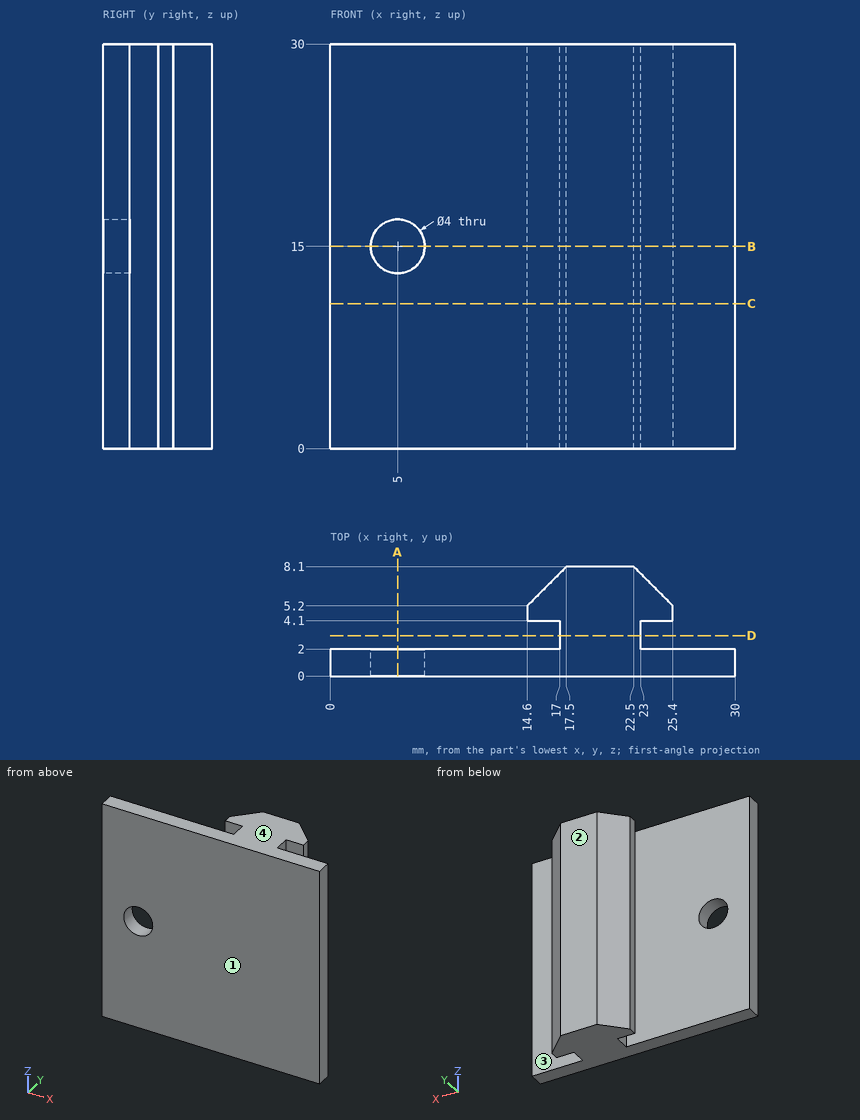
Study the drawing (mm; zero at the part's minimum x, y, z) and answer. Give positions to 0.01 mm unless a question says otherwise; leave off trailing zeros. Loops run counter-clockwise (first coordinate to the right, second up) from the corner with the lowest first, then second, coordinate; pieces in that order, holes last. Notation, with made-up numbers: M -6.5,-37.5 L 33.5,-37.5 A30 ccw 33.5,-12.5 Z; hole C -0.75,12 d7. An arc over 180 degrees is marked long. One line per item, written item: value. Start each with the question number.
1. Find section A-A (x = 5). Give the vertices of the cut face in (y, z).
2. Each of these flat-tipped pins is pushed along its axis until it touches: P1, Ø1.2, axis at y = 4.5, z = 9.5, coming from the -X side; P2, Ø5, axis at x = 5, z = 21, coming from the +Y side; P3, Ø0.6, axis at y = 3, z = 21.5, coming from the +X side. Where does it stop, or does it pass through?
3. Find section B-B (z = 15). Give the vertices of the cut face in (x, y), and give its area (3 significant figures).
4. Find the intervals of material crossed by probe 1 along Z at (x, y) = (5, 1.25); probe 2 along X at (y, z) = (1.3, 15); probe 3 along X at (y, z) = (4.5, 26.25), in increasing order.
5. Find section D-D (y = 3). Give the vertices of the cut face in (x, z).
6. Find section C-C (z = 10.75). Give the vertices of the cut face in (x, y).
7. Determine the mould class of the marked faces 1, 2, 3 and 4 for opening direction Y: released by +Y, released by -Y, zero draft, split by the parting line, or undercut.
Reported:
1. outline: M 0,0 L 2,0 L 2,13 L 0,13 Z; M 0,17 L 2,17 L 2,30 L 0,30 Z
2. P1: stops at x = 14.6
2. P2: stops at y = 2
2. P3: stops at x = 23
3. outline: M 0,0 L 3,0 L 3,2 L 0,2 Z; M 7,0 L 30,0 L 30,2 L 23,2 L 23,4.1 L 25.4,4.1 L 25.4,5.2 L 22.5,8.1 L 17.5,8.1 L 14.6,5.2 L 14.6,4.1 L 17,4.1 L 17,2 L 7,2 Z
3. area: 99.4 mm²
4. probe 1: z = 0 to 13, 17 to 30
4. probe 2: x = 0 to 3, 7 to 30
4. probe 3: x = 14.6 to 25.4
5. outline: M 17,0 L 23,0 L 23,30 L 17,30 Z
6. outline: M 0,0 L 30,0 L 30,2 L 23,2 L 23,4.1 L 25.4,4.1 L 25.4,5.2 L 22.5,8.1 L 17.5,8.1 L 14.6,5.2 L 14.6,4.1 L 17,4.1 L 17,2 L 0,2 Z
7. face 1: released by -Y
7. face 2: released by +Y
7. face 3: undercut
7. face 4: zero draft
